Geometry check sheet. Reference: the model listing, model coordinates, mm. A direction names the side the tool comes from. Round coordinates to 2 decimals unless told otherwise and drop trailing zeros. Write each loop counter-clockwise with the first axis right and the second up, starting at its lowest first coordinate (ties: lowest second). Pieces come first, ordered by that corner, then holes. Notation, with made-up numbers: M 89.5,72 L 100.5,72 A12 cw 100.5,85 Z; hole C 30,61.5 d10. An arc over 180 degrees is marked long. One line per item, written item: value. Start each with the question number.
1. Section check A-A (z = -194). Record the boundary of the cut face in (x, y) (3 decimals).
2. Release check for a two-part mould opening along X. For faces 6 (the flat face through (-133, 30.48, -143)), 7 (the flat face through (-3.76, 3.86, -112.7)), 8 (the flat face through (-101, 15, -25.4)), 9 (the flat face through (-13, 19, -190.5)) record: pulls with the +X half, pulls with the -X half, needs draft (parallel to the pull), parting line crosses it, or undercut.
3. Depth check by flat-ended pin: P1, Ø2, axis at x = -178, y = 7, coming from the -Z side; P2, Ø15, axis at x = -100, y = 8, coming from the -Z side; P3, Ø2, axis at y = 6, z = -107.5, coming from the -X side; P4, Ø11.5, axis at x = -12.68, y = 19.05, coming from the -Z side. Enter the tip coordinate at first touch or a pass-through.
4. Section check C-C (z = -55). Record the boundary of the cut face in (x, y).
5. Section check D-D (z = -12.7). Record the boundary of the cut face in (x, y) (3 decimals), and give its area (3 significant figures).
6. Section check B-B (y = 19.05). Record the boundary of the cut face in (x, z) (3 decimals).
7. Access from +Z, -Z, +X, -X, +Y, -Y to the whole of each face (thin tool, end or side, straight path). Record for faces 1 (the flat face through (-203, 15, -25.4)), 2 (the cylindrical face through (-209.82, 9.75, -14.76)), 3 (the flat face through (-50.8, 34, -128)), 4 (the flat face through (-76.2, 15, -126)), 5 (the flat face through (-45, 38.1, -94)).
8. Scan lines: probe 1 along X at (y, z) = (21.5, -80); probe 2 along X at (y, z) = (19.5, -215.5); probe 3 along Y at (x, z) = (-209, -12.7) (3 decimals). Record each from-to range of solid material in increasing order. Write a range as [from, to].
from build123d import *

# Parameters (mm, degrees)
SKETCH1_W           = 50.8
SKETCH1_H           = 203.2
BOSS_EXTRUDE1_DEPTH = 38.1
SKETCH3_R           = 9.525
CUT_EXTRUDE1_DEPTH  = 38.1
SKETCH4_R           = 9.525
CUT_EXTRUDE2_DEPTH  = 38.1
CUT_EXTRUDE3_DEPTH  = 7.62
CHAMFER1_SIZE       = 7.62


with BuildPart() as part:
    # Sketch1 → Boss-Extrude1 (new body)
    with BuildSketch(Plane(origin=(0, 0, 0), x_dir=(1, 0, 0), z_dir=(0, 1, 0))):
        Polygon((-25.4, 228.6), (-25.4, 25.4), (-76.2, 25.4), (-127, 25.4), (-177.8, 25.4), (-228.6, 25.4), (-228.6, 0), (0, 0), (0, 228.6), align=None)
        with Locations((-50.8, 127)):
            Rectangle(SKETCH1_W, SKETCH1_H)
        with Locations((-152.4, 127)):
            Rectangle(SKETCH1_W, SKETCH1_H)
    extrude(amount=BOSS_EXTRUDE1_DEPTH)

    # Sketch3 → Cut-Extrude1 (cut)
    with BuildSketch(Plane.ZY.offset(228.6)):
        with Locations((-12.7, 19.05)):
            Circle(SKETCH3_R)
    extrude(amount=-CUT_EXTRUDE1_DEPTH, mode=Mode.SUBTRACT)

    # Sketch4 → Cut-Extrude2 (cut)
    with BuildSketch(Plane(origin=(0, 0, -228.6), x_dir=(-1, 0, 0), z_dir=(0, 0, -1))):
        with Locations((12.684892179, 19.05)):
            Circle(SKETCH4_R)
    extrude(amount=-CUT_EXTRUDE2_DEPTH, mode=Mode.SUBTRACT)

    # Sketch5 → Cut-Extrude3 (cut)
    with BuildSketch(Plane(origin=(0, 38.1, 0), x_dir=(1, 0, 0), z_dir=(0, 1, 0))):
        Polygon((-50.8, 25.4), (-279.4, 25.371028997), (-279.4, 279.4), (-50.8, 279.4), align=None)
    extrude(amount=-CUT_EXTRUDE3_DEPTH, mode=Mode.SUBTRACT)

    # Chamfer1
    chamfer1_edges = [part.edges().sort_by_distance(p)[0] for p in [
        (0, 0, -114.3),
        (-114.3, 0, 0),
        (-114.3, 38.1, 0),
        (0, 38.1, -114.3),
    ]]
    chamfer(chamfer1_edges, length=CHAMFER1_SIZE)


solid = part.part
Result sheet:
1. outline: M -177.8,0 L -127,0 L -127,30.48 L -177.8,30.48 Z; M -76.2,0 L -7.62,0 L 0,7.62 L 0,30.48 L -7.62,38.1 L -50.8,38.1 L -50.8,30.48 L -76.2,30.48 Z; hole C -12.685,19.05 d19.05
2. face 6: needs draft
2. face 7: pulls with the +X half
2. face 8: undercut
2. face 9: undercut
3. P1: stops at z = -228.6
3. P2: stops at z = -25.4
3. P3: stops at x = -177.8
3. P4: stops at z = -190.5
4. outline: M -177.8,0 L -127,0 L -127,30.48 L -177.8,30.48 Z; M -76.2,0 L -7.62,0 L 0,7.62 L 0,30.48 L -7.62,38.1 L -50.8,38.1 L -50.8,30.48 L -76.2,30.48 Z
5. outline: M -228.6,0 L -7.62,0 L 0,7.62 L 0,30.48 L -7.62,38.1 L -228.6,38.1 L -228.6,28.575 L -190.5,28.575 L -190.5,9.525 L -228.6,9.525 Z
5. area: 7,930 mm2
6. outline: M -228.6,-25.4 L -177.8,-25.4 L -177.8,-228.6 L -127,-228.6 L -127,-25.4 L -76.2,-25.4 L -76.2,-228.6 L -22.21,-228.6 L -22.21,-190.5 L -3.16,-190.5 L -3.16,-228.6 L 0,-228.6 L 0,0 L -228.6,0 L -228.6,-3.175 L -190.5,-3.175 L -190.5,-22.225 L -228.6,-22.225 Z
7. face 1: -Z, -X, +Y, -Y
7. face 2: -X
7. face 3: -Z, -X, +Y
7. face 4: -Z, +Y, -Y
7. face 5: +Z, -Z, +X, -X, +Y
8. probe 1: x = [-177.8, -127], [-76.2, 0]
8. probe 2: x = [-177.8, -127], [-76.2, -22.2], [-3.17, 0]
8. probe 3: y = [0, 9.525], [28.575, 38.1]
